Autodesk Inventor part; units mm, degrees
ref_plane "YZ Plane" through (0, 0, 0) normal (1, 0, 0) x (0, 1, 0)
ref_plane "XZ Plane" through (0, 0, 0) normal (0, 1, 0) x (-1, 0, 0)
ref_plane "XY Plane" through (0, 0, 0) normal (0, 0, 1) x (1, 0, 0)
sketch "Boceto1" plane through (0, 0, 0) normal (0, 1, 0) x (-1, 0, 0)
  line L0 (-16.5612, -12.9032) -> (16.5612, -12.9032)
  line L1 (16.5612, -12.9032) -> (16.5612, 12.9032)
  line L2 (16.5612, 12.9032) -> (-16.5612, 12.9032)
  line L3 (-16.5612, 12.9032) -> (-16.5612, -12.9032)
  line L4 (-16.5612, -12.9032) -> (16.5612, 12.9032) construction
  line L5 (16.5612, -12.9032) -> (-16.5612, 12.9032) construction
  point P0 (0, 0)
  dimension "d0" = 16.5612
  dimension "d1" = 12.9032
extrude "Extrusión1" add sketch "Boceto1" along normal blind 1.27
sketch "Boceto2" plane through (-16.5612, 0, 12.9032) normal (0, 0, 1) x (1, 0, 0)
  line L0 (0, 1.27) -> (0, 35.1613)
  line L1 (0, 35.1613) -> (33.1216, 35.1613)
  line L2 (33.1216, 35.1613) -> (33.1216, 22.4613)
  line L3 (33.1216, 22.4613) -> (16.5608, 22.4613)
  line L4 (16.5608, 22.4613) -> (16.5612, 1.27)
  line L5 (33.1224, 1.27) -> (0, 1.27)
  point P0 (16.5612, 0)
  dimension "d4" = 33.1216
  dimension "d5" = 12.7
  dimension "d6" = 16.5608
  dimension "d7" = 21.1913
extrude "Extrusión2" add sketch "Boceto2" against normal blind 1.27
mirror "Simetría1" about plane through (0, 0, 0) normal (0, 0, 1) of "Extrusión2"
sketch "Boceto3" plane through (-0.0004, 22.4613, -11.6332) normal (1, 0, 0) x (0, 0, -1)
  line L0 (0, -21.191) -> (-23.2664, -21.191)
  line L1 (-23.2664, -21.191) -> (-23.2664, -0.0276)
  line L2 (-23.2664, -0.0276) -> (0, -0.0276)
  line L3 (0, 0) -> (0, -21.1913)
  line L4 (0, -0.0276) -> (0, -21.1913)
  line L5 (0, -21.1913) -> (-23.2664, -21.191)
  point P0 (-11.6332, -22.4613)
  dimension "d10" = 21.1634
extrude "Extrusión3" add sketch "Boceto3" against normal blind 1.27
sketch "Boceto4" plane through (-0.0004, 22.4337, 11.6332) normal (0, 1, 0) x (1, 0, 0)
  line L0 (16.561, 23.2664) -> (16.5608, 23.2664)
  line L1 (16.561, -1.27) -> (-1.2701, -1.27)
  line L2 (-1.27, 0) -> (-1.27, 23.2664)
  line L3 (-1.2701, -1.27) -> (-1.2701, 24.5364)
  line L4 (16.5612, 24.5364) -> (-16.5612, 24.5364)
  line L5 (-1.2701, 24.5364) -> (16.5612, 24.5364)
  line L6 (16.5612, 24.5364) -> (16.561, -1.27)
  dimension "d23" = 17.8312
extrude "Extrusión4" add sketch "Boceto4" along normal blind 1.27
sketch "Boceto7" plane through (16.5606, 22.434, 12.9032) normal (1, 0, 0) x (0, 0, -1)
  line L0 (0, 0) -> (25.8062, 0)
  line L1 (25.8062, -22.4334) -> (25.8062, 12.7279)
  line L2 (25.8062, 12.7279) -> (0, 12.7279)
  line L3 (0, 12.7279) -> (0, 0)
  line L4 (0, 1.27) -> (25.8064, 1.27)
  dimension "d28" = 1.27
  dimension "d29" = 25.8062
extrude "Extrusión7" add sketch "Boceto7" against normal blind 1.27
sketch "Boceto8" plane through (16.5606, 22.434, 12.9032) normal (1, 0, 0) x (0, 0, -1)
  line L0 (6.1467, 9.3592) -> (17.78, 9.3592)
  line L1 (17.78, 9.3592) -> (17.78, 4.572)
  line L2 (17.78, 4.572) -> (6.1467, 4.572)
  line L3 (6.1467, 4.572) -> (6.1467, 9.3592)
  line L4 (25.8064, 0) -> (0, 0)
  line L5 (0, 12.7273) -> (0, 1.27)
  point P0 (12.9031, -22.4337)
  dimension "d30" = 4.7871
  dimension "d31" = 11.6333
  dimension "d36" = 4.572
  dimension "d37" = 17.78
extrude "Extrusión8" cut sketch "Boceto8" against normal up to next
sketch "Boceto9" plane through (-0.0004, 22.4337, 11.6332) normal (0, -1, 0) x (1, 0, 0)
  circle A0 centre (8.2804, -3.5112) radius 2.3532
  line L0 (0, -24.5364) -> (0, 1.27)
  line L1 (15.291, 0) -> (-1.2701, 0)
  point P0 (0, -11.6332)
  dimension "d42" = 4.7064
  dimension "d43" = 8.2804
  dimension "d44" = 3.5112
extrude "Extrusión9" cut sketch "Boceto9" against normal up to next
sketch "Boceto10" plane through (0, 1.27, 12.9032) normal (1, 0, 0) x (0, 0, -1)
  circle A0 centre (23.114, 10.5788) radius 1.0858
  circle A1 centre (20.574, 10.5788) radius 1.0858
  line L0 (0, -0.0003) -> (25.8064, -0.0003)
  line L1 (0, 21.1637) -> (0, 0)
  point P0 (12.9032, -1.27)
  dimension "d47" = 2.1716
  dimension "d48" = 10.5791
  dimension "d49" = 23.114
  dimension "d50" = 2.54
  dimension "d51" = 10.5791
extrude "Extrusión10" cut sketch "Boceto10" against normal up to next
properties part number "sanicav"
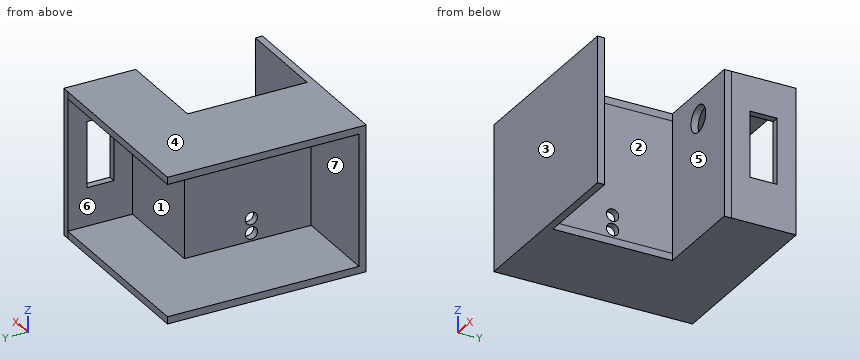
Work out the finished part from the listing and answer in its coordinate system (mm). Face numbers are marked on the shaded views. A direction names the side the tool comes from. Round coordinates to 2 decimals unless told otherwise and drop trailing zeros. Loops run counter-clockwise (first coordinate to the right, second up) from the corner with the lowest first, then second, coordinate; pieces in that order, holes last. Notation, with made-up numbers: M 70.5,32 L 126.5,32 A10 ccw 126.5,44 Z; hole C 22.5,29 d3. An arc over 180 degrees is marked long. One line per question, with ' | ' between items. Start each with the question number.
(1) Flat-ended cylindrical pins translate along their axes: pin 1 Ø0.6 at (y, z) = (11.5, 12) entering from +X; pin 2 Ø8 at (y, z) = (30.5, 6.5) entering from -X; pin 3 Ø11 at (y, z) = (13, 0.5) entering from -X. Find the tip coordinate at first contact, or state that the pin passes through.
(2) For a pull along Z with two mould halves and no side action, classify the marked faces 4, 5, 6 and 7 as released by +Z, released by -Z, zero draft, split by the parting line, or undercut.
(3) A tool of negligible diameter and unlimited length cuts with its end or side. For the marked faces 1, 2 and 3, from which of +Z, -Z, +X, -X, +Y, -Y can it reach the whole face along a straight path? Write none if from no direction.
(4) A cutting plane is placed at B-B on x = 8.28. Write down the section's boundary in (y, z), plus the area to 3 significant figures.
(5) A cutting plane is placed at A-A on x = 3. Write down the section's boundary in (y, z), plus the area to 3 significant figures.
(6) A cutting plane is placed at D-D on z = 1.75. Give the number of separate pieces and of enclosed holes in the cut face, plus the area to 3 significant figures.
(7) Find the intervals of material crossed by line 1 (Y direction, x = 12.5, z = 8); line 2 (Z direction, x = 12.5, y = 31); line 3 (X direction, y = 14, z = -3.5), in increasing order.
Geometry check:
1) pin 1: stops at x = 0 | pin 2: stops at x = 15.29 | pin 3: stops at x = -1.27
2) face 4: released by +Z | face 5: zero draft | face 6: undercut | face 7: undercut
3) face 1: -X, +Y | face 2: +Z, -Z, +X | face 3: +Z, -Z, +X, -X, -Y
4) outline: M 0,-12.9 L 1.27,-12.9 L 1.27,12.9 L 0,12.9 Z; M 22.43,-12.9 L 35.16,-12.9 L 35.16,-11.63 L 23.7,-11.63 L 23.7,5.77 L 22.43,5.77 Z; M 22.43,10.48 L 23.7,10.48 L 23.7,11.63 L 35.16,11.63 L 35.16,12.9 L 22.43,12.9 Z | area: 88.7 mm²
5) outline: M 0,-12.9 L 1.27,-12.9 L 1.27,12.9 L 0,12.9 Z; M 22.43,-12.9 L 35.16,-12.9 L 35.16,-11.63 L 23.7,-11.63 L 23.7,11.63 L 35.16,11.63 L 35.16,12.9 L 22.43,12.9 Z | area: 94.7 mm²
6) separate pieces: 3 | enclosed holes: 0 | area: 100 mm²
7) line 1: y = 0 to 1.27, 22.43 to 23.7 | line 2: z = -12.9 to -11.63, 11.63 to 12.9 | line 3: x = -1.27 to 0
